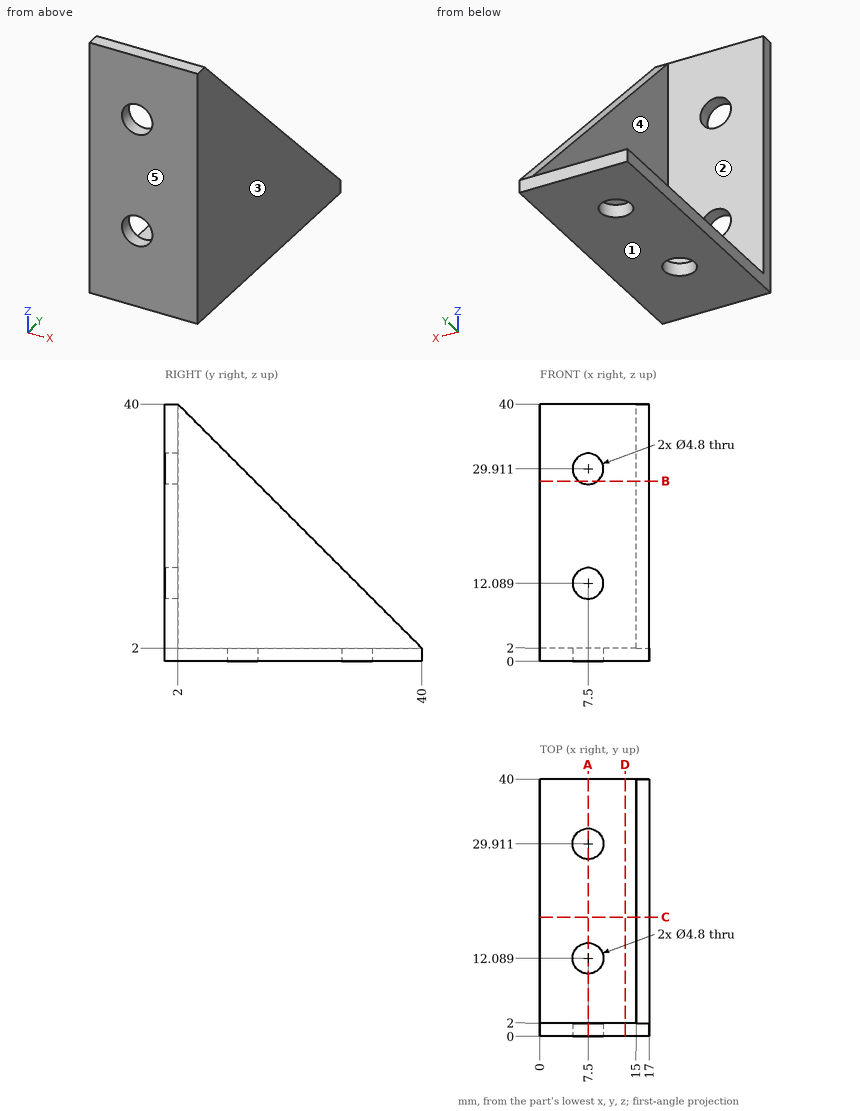
For this review, use the dimensioned drawing (mm, ordinates from the lowest corner) and the shaded views. A direction names the side the tool comes from. Round coordinates to 2 decimals unless told otherwise and drop trailing zeros. Write each loop counter-clockwise with the first axis right and the second up, starting at its lowest first coordinate (ties: lowest second). Pieces come first, ordered by that corner, then holes. Notation, with made-up numbers: M 85,-22.75 L 132,-22.75 A10 cw 132,-9.75 Z; hole C 8,-12 d3. An arc over 180 degrees is marked long. Write item = value, one per line. Start each with the question number.
(1) For the marked faces 1 and 2, list the 3-axis set-ups (+Z, -Z, +X, -X, +Y, -Y) from which the entire face can be reached by the end or side of a thin tool; tool diameter is ignored.
(2) We need section D-D (x = 13.25). Give the boundary of the cut face in (y, z).
(3) For line 1 along Z through (x, y) = (7.5, 1.5); line 2 along Y through (x, z) = (11, 11), list the stretches that pass through material, from the lowest coordinate up.
(4) We need section B-B (z = 28). Give the boundary of the cut face in (x, y), then the cut area to 3 significant figures.
(5) We need section A-A (x = 7.5). Give the boundary of the cut face in (y, z).
(6) We need section C-C (y = 18.5). Give the boundary of the cut face in (x, z), then the cut area to 3 significant figures.
(7) Clearance check with flat-ended pins moving along their axes: pin 1 Ø4.5 at (x, z) = (10.5, 16.5) entering from +Y; pin 2 Ø7.5 at (x, y) = (7.5, 12.09) entering from +Z; pin 3 Ø5 at (x, z) = (4.5, 33.5) entering from -Y; pin 4 Ø3 at (y, z) = (15, 14) entering from -X. State where each tip first meets the part, or that it passes through.
(8) The part is to be moulded in two halves that separate along X. For the marked faces 3, 4 and 5, say which applies: +X half, -X half, draft (parallel to the pull), parting line (faces both ways), or undercut.
Results found:
q1.face_1 = -Z, +X, -X, +Y, -Y
q1.face_2 = +Z, -X, +Y
q2.outline = M 0,0 L 40,0 L 40,2 L 2,2 L 2,40 L 0,40 Z
q3.line_1 = 0 to 9.69, 14.49 to 27.51, 32.31 to 40
q3.line_2 = 0 to 2
q4.outline = M 0,0 L 6.05,0 L 6.05,2 L 0,2 Z; M 8.95,0 L 17,0 L 17,14 L 15,14 L 15,2 L 8.95,2 Z
q4.area = 52.2 mm²
q5.outline = M 0,0 L 9.69,0 L 9.69,2 L 2,2 L 2,9.69 L 0,9.69 Z; M 0,14.49 L 2,14.49 L 2,27.51 L 0,27.51 Z; M 0,32.31 L 2,32.31 L 2,40 L 0,40 Z; M 14.49,0 L 27.51,0 L 27.51,2 L 14.49,2 Z; M 32.31,0 L 40,0 L 40,2 L 32.31,2 Z
q6.outline = M 0,0 L 17,0 L 17,23.5 L 15,23.5 L 15,2 L 0,2 Z
q6.area = 77.0 mm²
q7.pin_1 = 2
q7.pin_2 = 2
q7.pin_3 = 0
q7.pin_4 = 15
q8.face_3 = +X half
q8.face_4 = -X half
q8.face_5 = draft
